from build123d import *

# Parameters (mm, degrees)
CIRPATTERN1_COUNT = 4
CHAMFER1_SIZE     = 1.524


with BuildPart() as part:
    # Sketch1 → Body (revolve)
    with BuildSketch(Plane.XY):
        Polygon((-12.7, -38.416258567), (-10.16, -38.416258567), (-3.884, -8.89), (-3.884, -6.35), (-6.985, 0), (-9.525, 0), (-9.525, -3.81), (-7.366, -3.81), (-7.366, -6.19125), (-9.525, -6.19125), (-9.525, -15.24), (-7.773734167, -15.24), align=None)
    revolve(axis=Axis((0, 0, 0), (0, -1, 0)))

    # Sketch4 → SetScrew (revolve, cut)
    with BuildSketch(Plane(origin=(-9.525, -10.63625, 0), x_dir=(0, 0, 1), z_dir=(0, 1, 0))):
        Polygon((0, 0), (0, 2.54), (2.4892, 1.044337747), (2.4892, 0), align=None)
    setscrew = revolve(axis=Axis((-15.875, -10.63625, 0), (1, 0, 0)), mode=Mode.SUBTRACT)

    # CirPattern1: SetScrew ×4 about axis
    cirpattern1_axis = Axis((0, 0, 0), (0, 1, 0))
    for i in range(1, CIRPATTERN1_COUNT):
        add(setscrew.rotate(cirpattern1_axis, i * 360 / CIRPATTERN1_COUNT), mode=Mode.SUBTRACT)

    # Chamfer1
    chamfer1_edges = [part.edges().sort_by_distance(p)[0] for p in [
        (9.525, -3.81, 0),
        (9.525, -15.24, 0),
    ]]
    chamfer(chamfer1_edges, length=CHAMFER1_SIZE)


solid = part.part
Model file for the job. Use its own axes, mm. A direction names the side the tool comes from. Give positions to 0.01 mm unless a question says otherwise; leave off trailing zeros. Order: outer loops, then holes, each group sorted by start corner. A loop starts at its lowest first (then second) coordinate and runs counter-clockwise, first axis right, second up. Notation, with made-up numbers: (57, 55.5) - (85, 55.5) arc R16 ccw to (85, 78.5) - close; hole circle Ø9 at (29.25, 57). An arc over 180 degrees is marked (long way). Return JSON: item names as keys, results as strings.
1) Cut at A-A, the plane y = -34. Give the cut face in (x, z).
Geometry says:
{"outline": "circle Ø23.52 at (0, 0); hole circle Ø18.44 at (0, 0)"}
2) Cut at B-B, the plane y = -25.5. Give the cut face in (x, z).
Geometry says:
{"outline": "circle Ø19.91 at (0, 0); hole circle Ø14.83 at (0, 0)"}
3) 3-axis set-ups, long thin cutter, end or side, ignore diameter. For faces 1 (the cylindrical face through (-8.8, -10.01, 3.65)), 2 (the cylindrical face through (-3.399, -5.017, 6.535)), 3 (the cylindrical face through (8.89, -8.43, -1.15)): which of +Z, -Z, +X, -X, +Y, -Y reach the whole face in a straight line?
Geometry says:
{"face 1": "+Y", "face 2": "none", "face 3": "+X"}
4) Flat gauge pins, fed straight in: P1, Ø1.5, axis at x = 3.5, y = -11.5, coming from the -Z side; P2, Ø1.5, axis at x = 9.5, y = -10.5, coming from the +Z side; P3, Ø6.5, axis at y = -10.64, z = 0, coming from the +X side (3 decimals); P4, Ø1, axis at x = 0.5, z = 3, coming from the +Y side. Where does each tip first touch, or does it go through?
Geometry says:
{"P1": "z = -9.12", "P2": "z = 3.76", "P3": "x = 9.525", "P4": "through"}
5) Pull direction Z, two halves, no side cores. Call faces 4 (the conical face through (-6.656, -23.446, -2.096)), 5 (the conical face through (2.108, -24.415, 9.493)), 6 (the flat face through (6, -38.416, -9)): pulls with the +Z half, pulls with the -Z half, needs draft (parallel to the pull), parting line crosses it, or undercut.
Geometry says:
{"face 4": "undercut", "face 5": "parting line crosses it", "face 6": "needs draft"}
6) Probe line 1 (Z direction, x = 0, y = -6.9) (3 decimals); line 2 (Z direction, x = -4, y = -3). List the from-to ranges inside material, lowest first. Write a range as from..to.
Geometry says:
{"line 1": "-9.525..-3.884, 3.884..9.525", "line 2": "-7.85..-3.8, 3.8..7.85"}
